Source: CAD feature listing. Evaluate the final solid. Frame: model axes, mm. Face numbers are marked on the shaded views. Give positions to 0.01 mm unless a question says otherwise; leave off trailing zeros. Order: outer loops, then holes, each group sorted by start corner. A loop starts at its lowest first (then second) coordinate and runs counter-clockwise, first axis right, second up. Notation, with made-up numbers: (72.25, 76.25) - (78.25, 76.25) arc R13 cw to (78.25, 101.25) - close; hole circle Ø7 at (77.25, 29). An arc over 180 degrees is marked (long way). Write each question's results on one line, items separated by ' | '. Start each with the question number.
Item 1: Mould query, pull axis Z, two halves, no side actions, for the marked faces 1 and 2. Classes: released by +Z, released by -Z, zero draft, split by the parting line, or undercut.
Item 2: Section B-B on x = 3.75. Output: boundary loops of the cut face in (y, z), and give its area (3 significant figures).
Item 3: Contact query for flat-ended pins moving along their axis: pin 1 Ø1 at (y, z) = (0, 7) entering from +X; pin 2 Ø1 at (x, z) = (-3.5, -8) entering from +Y. Output: stop coordinate, or through.
Item 4: Section C-C on y = -0.5. Output: boundary loops of the cut face in (x, z), and give its area (3 significant figures).
Item 5: Line query: line 1 along Z through (x, y) = (0, 0.6); line 2 along X through (y, z) = (0.95, 6.5); line 3 along X through (y, z) = (-0.2, -10). Output: solid intervals per line, ascending.
Item 6: Section D-D on x = -3.5. Output: boundary loops of the cut face in (y, z).
Item 7: Section A-A on x = 0. Output: boundary loops of the cut face in (y, z), and give its area (3 significant figures).
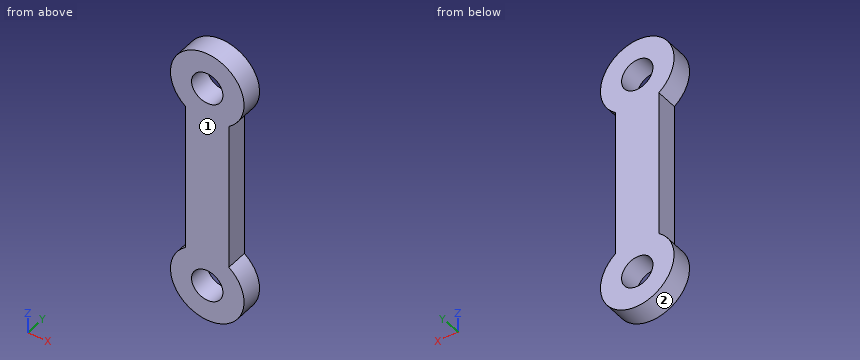
Autodesk Inventor part; units mm, degrees
ref_plane "YZ Plane" through (0, 0, 0) normal (1, 0, 0) x (0, 1, 0)
ref_plane "XZ Plane" through (0, 0, 0) normal (0, 1, 0) x (-1, 0, 0)
ref_plane "XY Plane" through (0, 0, 0) normal (0, 0, 1) x (1, 0, 0)
sketch "Sketch1" plane through (0, 0, 0) normal (0, 1, 0) x (-1, 0, 0)
  line L0 (2.54, 10.414) -> (-2.54, 10.414)
  line L1 (-2.54, 10.414) -> (-2.54, -10.414)
  line L2 (-2.54, -10.414) -> (2.54, -10.414)
  line L3 (2.54, -10.414) -> (2.54, 10.414)
  circle A0 centre (0, 12.2555) radius 1.8415
  circle A1 centre (0, -12.2555) radius 1.8415
  circle A2 centre (0, -12.2555) radius 4.318
  circle A3 centre (0, 12.2555) radius 4.318
  point P0 (0, 0)
  point P1 (0, 10.414)
  point P2 (0, -10.414)
  dimension "d6" = 3.683
  dimension "d0" = 10.414
  dimension "d1" = 20.828
  dimension "d2" = 10.414
  dimension "d3" = 5.08
  dimension "d4" = 2.54
  dimension "d5" = 2.54
  dimension "d7" = 8.636
extrude "Extrusion1" add sketch "Sketch1" along normal blind 1.27 and the other way blind 1.27
properties part number "conneectors"
Evaluation:
1) face 1: zero draft | face 2: undercut
2) outline: (-1.27, -14.4) - (1.27, -14.4) - (1.27, -10.11) - (-1.27, -10.11) - close; (-1.27, 10.11) - (1.27, 10.11) - (1.27, 14.4) - (-1.27, 14.4) - close | area: 21.7 mm^2
3) pin 1: stops at x = 2.54 | pin 2: passes through
4) outline: (-2.54, -8.76) arc R4.32 ccw (long way) to (2.54, -8.76) - (2.54, 8.76) arc R4.32 ccw (long way) to (-2.54, 8.76) - close; hole circle Ø3.68 at (0, -12.26); hole circle Ø3.68 at (0, 12.26) | area: 179 mm^2
5) line 1: z = -16.57 to -14.1, -10.41 to 10.41, 14.1 to 16.57 | line 2: x = -2.54 to 2.54 | line 3: x = -3.68 to 3.68
6) outline: (-1.27, -14.78) - (1.27, -14.78) - (1.27, -9.73) - (-1.27, -9.73) - close; (-1.27, 9.73) - (1.27, 9.73) - (1.27, 14.78) - (-1.27, 14.78) - close
7) outline: (-1.27, -16.57) - (1.27, -16.57) - (1.27, -14.1) - (-1.27, -14.1) - close; (-1.27, -10.41) - (1.27, -10.41) - (1.27, 10.41) - (-1.27, 10.41) - close; (-1.27, 14.1) - (1.27, 14.1) - (1.27, 16.57) - (-1.27, 16.57) - close | area: 65.5 mm^2
